Input: dimensioned drawing with shaded views. Units: mm. Origin: part minimum x, y, z. A direction names the side the tool comes from. Round coordinates to 2 decimals unless told otherwise and drop trailing zeros. Order: outer loops, then holes, each group sorted by start corner. A loop starts at its lowest first (then second) coordinate and runs counter-clockwise, first axis right, second up. Notation, with made-up numbers: M 4.5,31.25 L 62.5,31.25 A35 ccw 62.5,63.25 Z; hole C 51.25,9 d7. An arc over 180 degrees is marked long. Use one line per item in the form item = value. Start each with the question number.
Q1. Reachability of the marked faces 1 and 2 from +Z, -Z, +X, -X, +Y, -Y: full face, straight path, thin tool, end or side. Return the list, or none.
Q2. Contact query for flat-ended pins moving along their axis: pin 1 (5 mm diameter, centred on x = 30.5, z = 16, fed in from +Y); pin 2 (2 mm diameter, centred on y = 18.5, z = 26.5, fed in from +X); pin 3 (4 mm diameter, centred on x = 8.5, y = 12.5, fed in from +Z). Output: stop coordinate, or through.
Q3. Section D-D (y = 2.25). Return the cut outline in (x, z).
Q4. Section B-B (z = 19.1). Return the cut outline in (x, y), plus the area to 3 significant figures.
Q5. Section C-C (y = 14.5). Return the cut outline in (x, z).
Q6. Material intervals for probe 1 along Y at (x, z) = (28, 29.5); probe 2 along Z at (x, y) = (19, 12.25); probe 3 along Y at (x, z) = (19.5, 13), sorted ascending.
Q7. Section A-A (x = 19.1). Return the cut outline in (y, z), plus the area to 3 significant figures.
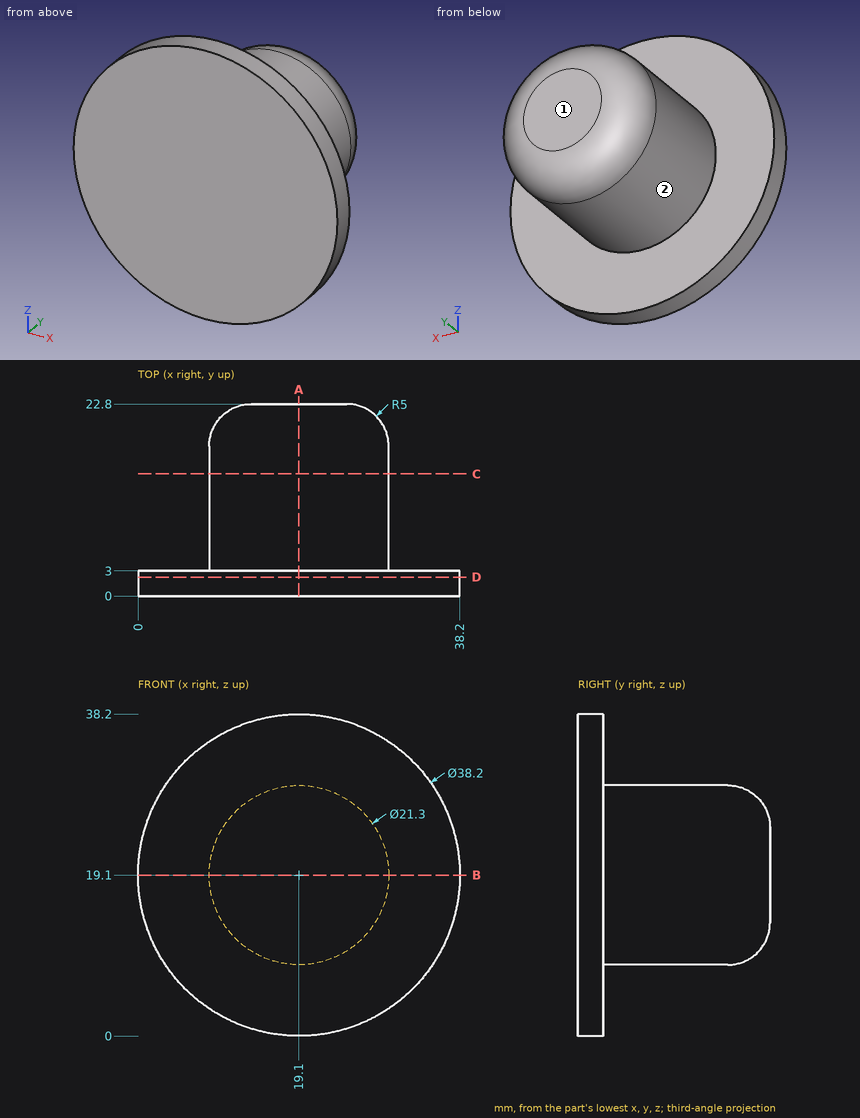
Results list:
q1.face_1 = +Z, -Z, +X, -X, +Y
q1.face_2 = +Y
q2.pin_1 = 21.2
q2.pin_2 = 27.57
q2.pin_3 = 25.38
q3.outline = C 19.1,19.1 d38.2
q4.outline = M 0,0 L 38.2,0 L 38.2,3 L 29.75,3 L 29.75,17.8 A5 ccw 24.75,22.8 L 13.45,22.8 A5 ccw 8.45,17.8 L 8.45,3 L 0,3 Z
q4.area = 526 mm2
q5.outline = C 19.1,19.1 d21.3
q6.probe_1 = 0 to 3
q6.probe_2 = 8.45 to 29.75
q6.probe_3 = 0 to 22.78
q7.outline = M 0,0 L 3,0 L 3,8.45 L 17.8,8.45 A5 ccw 22.8,13.45 L 22.8,24.75 A5 ccw 17.8,29.75 L 3,29.75 L 3,38.2 L 0,38.2 Z
q7.area = 526 mm2
